```python
from build123d import *

# Parameters (mm, degrees)
SKETCH1_W          = 3.5
SKETCH1_H          = 20
SKETCH1_W_2        = 0.351227394
SKETCH1_H_2        = 9.140463919
SKETCH3_R          = 0.848772606
CUT_EXTRUDE1_DEPTH = 8


with BuildPart() as part:
    # Sketch1 → Revolve1 (revolve)
    with BuildSketch(Plane.XY, mode=Mode.PRIVATE) as revolve1_sk:
        with Locations((-2.95, 10)):
            Rectangle(SKETCH1_W, SKETCH1_H)
        with Locations((-1.024386303, 15.429768041)):
            Rectangle(SKETCH1_W_2, SKETCH1_H_2)
    revolve(revolve1_sk.sketch.rotate(Axis((0, 0, 0), (0, 1, 0)), 270), axis=Axis((0, 0, 0), (0, 1, 0)))

    # Sketch3 → Cut-Extrude1 (cut)
    # profile 1 of 5: a face of its own
    with BuildSketch(Plane(origin=(0, 20, 0), x_dir=(1, 0, 0), z_dir=(0, 1, 0))):
        with BuildLine():
            Line((0.452879675, 1.43), (-0.452879675, 1.43))
            ThreePointArc((-0.452879675, 1.43), (-1.428365431, 0.458008946), (-1.2, -0.9))
            Line((-1.2, -0.9), (1.2, -0.9))
            ThreePointArc((1.2, -0.9), (1.428365431, 0.458008946), (0.452879675, 1.43))
        make_face()
        with Locations(Location((0, 0, 0), (0, 0, 90))):
            Circle(SKETCH3_R, mode=Mode.SUBTRACT)
    # profile 2 of 5: a face of its own
    with BuildSketch(Plane(origin=(0, 20, 0), x_dir=(1, 0, 0), z_dir=(0, 1, 0))):
        with BuildLine():
            ThreePointArc((0.452879675, 1.43), (0, 1.5), (-0.452879675, 1.43))
            Line((-0.452879675, 1.43), (0.452879675, 1.43))
        make_face()
    # profile 3 of 5: a face of its own
    with BuildSketch(Plane(origin=(0, 20, 0), x_dir=(1, 0, 0), z_dir=(0, 1, 0))):
        with BuildLine():
            ThreePointArc((0.717704675, 1.43), (0, 1.6), (-0.717704675, 1.43))
            Line((-0.717704675, 1.43), (-0.452879675, 1.43))
            ThreePointArc((-0.452879675, 1.43), (0, 1.5), (0.452879675, 1.43))
            Line((0.452879675, 1.43), (0.717704675, 1.43))
        make_face()
    # profile 4 of 5: a face of its own
    with BuildSketch(Plane(origin=(0, 20, 0), x_dir=(1, 0, 0), z_dir=(0, 1, 0))):
        with BuildLine():
            ThreePointArc((-0.717704675, 1.43), (-1.56307595, 0.341750749), (-1.2489996, -1))
            Line((-1.2489996, -1), (1.2489996, -1))
            ThreePointArc((1.2489996, -1), (1.56307595, 0.341750749), (0.717704675, 1.43))
            Line((0.717704675, 1.43), (0.452879675, 1.43))
            ThreePointArc((0.452879675, 1.43), (1.428365431, 0.458008946), (1.2, -0.9))
            Line((1.2, -0.9), (-1.2, -0.9))
            ThreePointArc((-1.2, -0.9), (-1.428365431, 0.458008946), (-0.452879675, 1.43))
            Line((-0.452879675, 1.43), (-0.717704675, 1.43))
        make_face()
    # profile 5 of 5: a face of its own
    with BuildSketch(Plane(origin=(0, 20, 0), x_dir=(1, 0, 0), z_dir=(0, 1, 0))):
        with Locations(Location((0, 0, 0), (0, 0, 90))):
            Circle(SKETCH3_R)
    extrude(amount=-CUT_EXTRUDE1_DEPTH, mode=Mode.SUBTRACT)


solid = part.part
```
The model under review builds one solid part; all positions refer to its coordinate system, in mm. A direction names the side the tool comes from. Round coordinates to 2 decimals unless told otherwise and drop trailing zeros. Loops run counter-clockwise (first coordinate to the right, second up) from the corner with the lowest first, then second, coordinate; pieces in that order, holes last. Notation, with made-up numbers: M 85,73.5 L 128,73.5 A21 cw 128,96.5 Z; hole C 32,21 d10. An arc over 180 degrees is marked long. Answer as a JSON object with one key per item and string values.
(1) Tool access review of faces 4 (the flat face through (0, 12, -1)), 5 (the flat face through (2, 20, 0)), 6 (the flat face through (0, 10.86, 1)): name each direction out of +Z, -Z, +X, -X, +Y, -Y from which nothing blocks a thin tool from reaching the whole face with its end or side.
Resolved:
{"face 4": "+Y", "face 5": "+Z, -Z, +X, -X, +Y", "face 6": "-Y"}
(2) Take a section at C-C on y = 10. Give the boundary of the cut face in (x, z), and give its area (3 significant figures).
Resolved:
{"outline": "C 0,0 d9.4; hole C 0,0 d2.4", "area": "64.9 mm²"}
(3) Take a section at B-B on z = 0. Give the boundary of the cut face in (x, y), and give its area (3 significant figures).
Resolved:
{"outline": "M -4.7,0 L -1.2,0 L -1.2,10.86 L -0.85,10.86 L -0.85,12 L -1.6,12 L -1.6,20 L -4.7,20 Z; M 0.85,10.86 L 1.2,10.86 L 1.2,0 L 4.7,0 L 4.7,20 L 1.6,20 L 1.6,12 L 0.85,12 Z", "area": "134 mm²"}
(4) Take a section at A-A on x = 0. Give the boundary of the cut face in (y, z).
Resolved:
{"outline": "M 0,-4.7 L 20,-4.7 L 20,-1.6 L 12,-1.6 L 12,-0.85 L 10.86,-0.85 L 10.86,-1.2 L 0,-1.2 Z; M 0,1.2 L 10.86,1.2 L 10.86,0.85 L 12,0.85 L 12,1 L 20,1 L 20,4.7 L 0,4.7 Z"}
(5) To check wall thickness, follow line 1 along X through (y, z) = (11.6, 0); line 2 along X through (y, z) = (8.75, 0); line 3 along Z through (x, y) = (0.5, 9.75). State the ranges of each line that lie inside material, in increasing order.
Resolved:
{"line 1": "-4.7 to -0.85, 0.85 to 4.7", "line 2": "-4.7 to -1.2, 1.2 to 4.7", "line 3": "-4.67 to -1.09, 1.09 to 4.67"}
(6) Clearance check with flat-ended pins moving along their axes: P1, Ø1, axis at x = -3, y = 5, coming from the -Z side; P2, Ø1.4, axis at x = 0, z = 0, coming from the +Y side; P3, Ø1, axis at y = 17.5, z = 3.5, coming from the -X side. State where each tip first meets the part, or that it passes through.
Resolved:
{"P1": "z = -3.98", "P2": "through", "P3": "x = -3.62"}
(7) Draft analysis for pull direction X (two halves, no side actions). For faces 1 (the cylindrical face through (-1.01, 5.51, -0.65)), 2 (the flat face through (1, 0, -1)), 3 (the cylindrical face through (-1.412, 10.14, -4.483)), state which applies: released by +X, released by -X, zero draft, split by the parting line, or undercut.
Resolved:
{"face 1": "undercut", "face 2": "zero draft", "face 3": "split by the parting line"}
(8) Take a section at D-D on x = 2.5. Give the boundary of the cut face in (y, z).
Resolved:
{"outline": "M 0,-3.98 L 20,-3.98 L 20,3.98 L 0,3.98 Z"}
